For this review, take the finished solid that the model builds, in its own axes (mm). Face numbers are marked on the shaded views. A direction names the side the tool comes from. Give positions to 0.01 mm unless a question says otherwise; leave off trailing zeros. Order: outer loops, then holes, each group sorted by start corner. A loop starts at its lowest first (then second) coordinate and runs counter-clockwise, first axis right, second up. Notation, with made-up numbers: M 84.25,0 L 130.25,0 A22 cw 130.25,18 Z; hole C 71,54 d10. An arc over 180 degrees is marked long. Use CSV: the item, a comma, the result in double quotes. Start each with the question number.
(1) Tool access review of the marked faces 1, 2 and 3: name each direction out of +Z, -Z, +X, -X, +Y, -Y from which nothing blocks a thin tool from reaching the whole face with its end or side.
(2) Consider section A-A (x = 47). Write out the cut boundary in (y, z).
(3) Consider section D-D (x = -8). Write out the cut boundary in (y, z), and give its area (3 significant figures).
(4) Clearance check with flat-ended pins moving along their axes: P1, Ø5.5, axis at y = 1.5, z = -18, coming from the -X side; P2, Ø22.5, axis at x = -16.5, z = -15, coming from the +Y side; P3, Ø1.5, axis at y = 2.5, z = -20.5, coming from the +X side. State where each tip first meets the part, or that it passes through.
(5) Wall thickness on L1, parallel to X at y = -7, z = -10.5; L2, parallel to X at y = -10, z = 5; L3, parallel to Y at x = -56, z = -24: over which ranges is each line inside the solid? List them lowest first. Write a range as from..to.
(6) Consider section B-B (y = -4). Write out the cut boundary in (x, z), and give its area (3 significant figures).
(7) Draft analysis for pull direction X (two halves, no side actions). For the marked faces 4, 5 and 6, state which applies: pulls with the +X half, pulls with the -X half, needs draft (parallel to the pull), parting line crosses it, or undercut.
(8) Consider section C-C (z = 18). Write out the cut boundary in (x, y).
```python
from build123d import *

# Parameters (mm, degrees)
SKETCH1_W           = 85
SKETCH1_H           = 80
BOSS_EXTRUDE1_DEPTH = 5
SKETCH4_W           = 5
SKETCH4_H           = 80
BOSS_EXTRUDE3_DEPTH = 30
SKETCH6_R           = 1.25
CUT_EXTRUDE3_DEPTH  = 101.249688279
SKETCH3_W           = 85
SKETCH3_H           = 80
BOSS_EXTRUDE4_DEPTH = 15
SKETCH8_W           = 8
SKETCH8_H           = 12
CUT_EXTRUDE4_DEPTH  = 69.053287944
MOVE_FACE1_BY       = 3
BOSS_EXTRUDE5_DEPTH = 18.5
BOSS_EXTRUDE6_START = -103.5
BOSS_EXTRUDE6_DEPTH = 18.5
CUT_EXTRUDE5_START  = -13
CUT_EXTRUDE5_DEPTH  = 13
CUT_EXTRUDE6_START  = -85
CUT_EXTRUDE6_DEPTH  = 13
DELETEFACE1_START   = 37.5
DELETEFACE1_DEPTH   = 23.5
DELETEFACE2_START   = -61
DELETEFACE2_DEPTH   = 23.5
DELETEFACE3_START   = -61
DELETEFACE3_DEPTH   = 122


# Read off the part's stored shape, not the designer's step: DeleteFace1, DeleteFace2, DeleteFace3
with BuildPart() as part:
    # Sketch1 → Boss-Extrude1 (new body)
    with BuildSketch(Plane(origin=(0, 0, 0), x_dir=(1, 0, 0), z_dir=(0, 1, 0))):
        Rectangle(SKETCH1_W, SKETCH1_H)
    extrude(amount=BOSS_EXTRUDE1_DEPTH)

    # Sketch4 → Boss-Extrude3 (add)
    with BuildSketch(Plane(origin=(0, 5, 0), x_dir=(1, 0, 0), z_dir=(0, 1, 0))):
        with Locations((-40, 0)):
            Rectangle(SKETCH4_W, SKETCH4_H)
        with Locations((40, 0)):
            Rectangle(SKETCH4_W, SKETCH4_H)
    extrude(amount=BOSS_EXTRUDE3_DEPTH)

    # Sketch6 → Cut-Extrude3 (cut, through all)
    with BuildSketch(Plane.ZY.offset(42.5)):
        with Locations((10.624581332, 2.504153155)):
            Circle(SKETCH6_R)
        with Locations((3.123107186, 18.591116375)):
            Circle(SKETCH6_R)
        Polygon((24.335207615, 35), (-40, 5), (-40, 35), align=None)
    extrude(amount=-CUT_EXTRUDE3_DEPTH, mode=Mode.SUBTRACT)

    # Sketch3 → Boss-Extrude4 (add)
    with BuildSketch(Plane.XZ):
        Rectangle(SKETCH3_W, SKETCH3_H)
        Polygon((29.5, -21.75), (37.5, -21.75), (37.5, -9.75), (29.5, -9.75), (29.5, 31.75), (-29.5, 31.75), (-29.5, -31.75), (29.5, -31.75), align=None, mode=Mode.SUBTRACT)
    extrude(amount=BOSS_EXTRUDE4_DEPTH)

    # Sketch8 → Cut-Extrude4 (cut, through all)
    with BuildSketch(Plane.XZ):
        with Locations((33.5, -15.75)):
            Rectangle(SKETCH8_W, SKETCH8_H)
    extrude(amount=-CUT_EXTRUDE4_DEPTH, mode=Mode.SUBTRACT)

    # Move Face1: a face moved outward by 3.0
    extrude(part.faces().sort_by_distance((0, -1.25, 40))[0], amount=MOVE_FACE1_BY, dir=(0, 0, 1))

    # Sketch7 → Boss-Extrude5 (add)
    with BuildSketch(Plane(origin=(42.5, 0, 0), x_dir=(0, 0, -1), z_dir=(1, 0, 0))):
        Polygon((40, -15), (40, 5), (-24.335207615, 35), (-43, 35), (-43, -15), align=None)
        with BuildLine():
            Line((-26.692544096, 32.64359903), (27.051507675, 7.582336108))
            Line((27.051507675, 7.582336108), (26.26502094, 1.163306695))
            Line((26.26502094, 1.163306695), (21.61622006, -8.806078963))
            Line((21.61622006, -8.806078963), (17.204502177, -13.534635329))
            Line((17.204502177, -13.534635329), (-36.539549595, 11.526627592))
            ThreePointArc((-36.539549595, 11.526627592), (-38.86638421, 14.065921988), (-38.716152458, 17.506794811))
            Line((-38.716152458, 17.506794811), (-36.962286672, 21.267972127))
            Line((-36.962286672, 21.267972127), (-41.493825607, 23.381063436))
            Line((-41.493825607, 23.381063436), (-38.958116037, 28.818910158))
            Line((-38.958116037, 28.818910158), (-34.426577102, 26.70581885))
            Line((-34.426577102, 26.70581885), (-32.672711316, 30.466996166))
            ThreePointArc((-32.672711316, 30.466996166), (-30.133416919, 32.793830782), (-26.692544096, 32.64359903))
        make_face(mode=Mode.SUBTRACT)
    extrude(amount=BOSS_EXTRUDE5_DEPTH)

    # Sketch7<2> → Boss-Extrude6 (add)
    with BuildSketch(Plane(origin=(42.5, 0, 0), x_dir=(0, 0, -1), z_dir=(1, 0, 0)).offset(BOSS_EXTRUDE6_START)):
        Polygon((40, -15), (40, 5), (-24.335207615, 35), (-43, 35), (-43, -15), align=None)
        with BuildLine():
            Line((-26.692544096, 32.64359903), (27.051507675, 7.582336108))
            Line((27.051507675, 7.582336108), (26.26502094, 1.163306695))
            Line((26.26502094, 1.163306695), (21.61622006, -8.806078963))
            Line((21.61622006, -8.806078963), (17.204502177, -13.534635329))
            Line((17.204502177, -13.534635329), (-36.539549595, 11.526627592))
            ThreePointArc((-36.539549595, 11.526627592), (-38.86638421, 14.065921988), (-38.716152458, 17.506794811))
            Line((-38.716152458, 17.506794811), (-36.962286672, 21.267972127))
            Line((-36.962286672, 21.267972127), (-41.493825607, 23.381063436))
            Line((-41.493825607, 23.381063436), (-38.958116037, 28.818910158))
            Line((-38.958116037, 28.818910158), (-34.426577102, 26.70581885))
            Line((-34.426577102, 26.70581885), (-32.672711316, 30.466996166))
            ThreePointArc((-32.672711316, 30.466996166), (-30.133416919, 32.793830782), (-26.692544096, 32.64359903))
        make_face(mode=Mode.SUBTRACT)
    extrude(amount=BOSS_EXTRUDE6_DEPTH)

    # Sketch9 → Cut-Extrude5 (cut)
    with BuildSketch(Plane(origin=(42.5, 0, 0), x_dir=(0, 0, -1), z_dir=(1, 0, 0)).offset(CUT_EXTRUDE5_START)):
        Polygon((21.61622006, -8.806078963), (26.26502094, 1.163306695), (27.051507675, 7.582336108), (19.597005499, 11.058427561), (9.75, -10.058543877), (17.204502177, -13.534635329), align=None)
    extrude(amount=CUT_EXTRUDE5_DEPTH, mode=Mode.SUBTRACT)

    # Sketch9<3> → Cut-Extrude6 (cut)
    with BuildSketch(Plane(origin=(42.5, 0, 0), x_dir=(0, 0, -1), z_dir=(1, 0, 0)).offset(CUT_EXTRUDE6_START)):
        Polygon((21.61622006, -8.806078963), (26.26502094, 1.163306695), (27.051507675, 7.582336108), (19.597005499, 11.058427561), (9.75, -10.058543877), (17.204502177, -13.534635329), align=None)
    extrude(amount=CUT_EXTRUDE6_DEPTH, mode=Mode.SUBTRACT)

    # DeleteFace1 outline → DeleteFace1 (add)
    with BuildSketch(Plane.YZ.offset(DELETEFACE1_START)):
        Polygon((43.703535627, 43), (35, 43), (35, 24.335207615), align=None)
    extrude(amount=DELETEFACE1_DEPTH)

    # DeleteFace2 outline → DeleteFace2 (add)
    with BuildSketch(Plane.YZ.offset(DELETEFACE2_START)):
        Polygon((43.703535627, 43), (35, 43), (35, 24.335207615), align=None)
    extrude(amount=DELETEFACE2_DEPTH)

    # DeleteFace3 outline → DeleteFace3 (add)
    with BuildSketch(Plane.YZ.offset(DELETEFACE3_START)):
        Polygon((-15, -82.89013841), (5, -40), (-15, -40), align=None)
    extrude(amount=DELETEFACE3_DEPTH)


solid = part.part
```
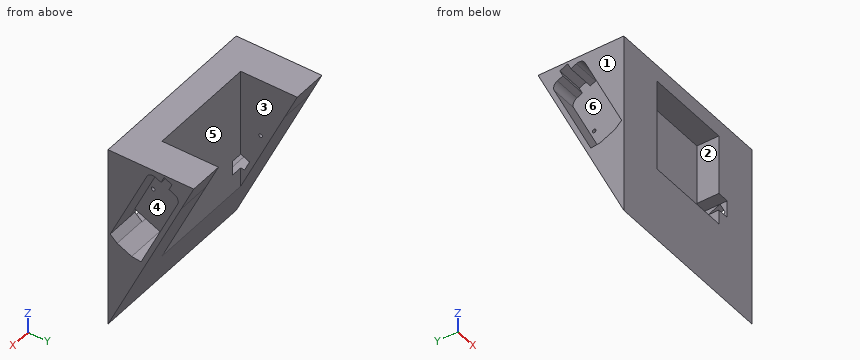
Check result:
1,face 1,"+Z, -Z, -X, +Y, -Y"
1,face 2,"-Y"
1,face 3,"+Z, -Z, +Y"
2,outline,"M -15,-82.89 L 43.7,43 L -15,43 Z; hole M -13.53,-17.2 L -8.81,-21.62 L 1.16,-26.27 L 7.58,-27.05 L 32.64,26.69 A4.5 ccw 30.47,32.67 L 26.71,34.43 L 28.82,38.96 L 23.38,41.49 L 21.27,36.96 L 17.51,38.72 A4.5 ccw 11.53,36.54 Z"
3,outline,"M -15,-82.89 L 5,-40 L 5,43 L -15,43 L -15,31.75 L 0,31.75 L 0,-31.75 L -15,-31.75 Z; hole C 2.5,10.62 d2.5"
3,area,"1,130 mm^2"
4,P1,"stops at x = -42.5"
4,P2,"stops at y = 5"
4,P3,"stops at x = 29.5"
5,L1,"x = -42.5..-29.5, 37.5..42.5"
5,L2,"x = -61..-29.5, 29.5..61"
5,L3,"y = -15..-3.69, 9.01..12.46"
6,outline,"M -61,-59.3 L 61,-59.3 L 61,-23.86 L 29.5,-23.86 L 29.5,-31.75 L -29.5,-31.75 L -29.5,-23.86 L -61,-23.86 Z; M -61,3.24 L -42.5,3.24 L -42.5,-12.58 L -29.5,-12.58 L -29.5,31.75 L 29.5,31.75 L 29.5,-9.75 L 37.5,-9.75 L 37.5,-12.58 L 42.5,-12.58 L 42.5,3.24 L 61,3.24 L 61,43 L -61,43 Z"
6,area,"7,420 mm^2"
7,face 4,"pulls with the +X half"
7,face 5,"undercut"
7,face 6,"pulls with the -X half"
8,outline,"M -61,-15 L -29.5,-15 L -29.5,0 L 29.5,0 L 29.5,-15 L 61,-15 L 61,2.88 L 42.5,2.88 L 42.5,28.59 L 61,28.59 L 61,32.05 L 37.5,32.05 L 37.5,5 L -37.5,5 L -37.5,32.05 L -61,32.05 L -61,28.59 L -42.5,28.59 L -42.5,2.88 L -61,2.88 Z"
